from build123d import *

# Parameters (mm, degrees)
SKETCH_2_R          = 55
EXTRUDE_1_DEPTH     = 15
SKETCH_3_R          = 50
CUT_EXTRUDE_1_DEPTH = 10
EXTRUDE_3_DEPTH     = 15
CUT_EXTRUDE_4_DEPTH = 10
CUT_EXTRUDE_5_DEPTH = 10
FILLET_1_R          = 5
FILLET_2_R          = 5
FILLET_3_R          = 5


with BuildPart() as part:
    # 草圖2 → 填料-伸長1 (new body)
    with BuildSketch(Plane(origin=(0, 0, 0), x_dir=(1, 0, 0), z_dir=(0, 1, 0))):
        with Locations(Location((0, 0, 0), (0, 0, 270))):
            Circle(SKETCH_2_R)
    extrude(amount=EXTRUDE_1_DEPTH)

    # 草圖3 → 除料-伸長1 (cut)
    with BuildSketch(Plane(origin=(0, 15, 0), x_dir=(1, 0, 0), z_dir=(0, 1, 0))):
        with Locations(Location((0, 0, 0), (0, 0, 270))):
            Circle(SKETCH_3_R)
    extrude(amount=-CUT_EXTRUDE_1_DEPTH, mode=Mode.SUBTRACT)

    # 草圖8 → 填料-伸長3 (add)
    with BuildSketch(Plane.XZ):
        with BuildLine():
            ThreePointArc((55, 0), (23.675491822, -49.643439516), (-34.617130436, -42.739376228))
            ThreePointArc((-34.617130436, -42.739376228), (6.919661262, -68.581943503), (55, -77.605489076))
            Line((55, -77.605489076), (55, 0))
        make_face()
        with BuildLine():
            ThreePointArc((-55, 0), (-38.890872965, 38.890872965), (0, 55))
            Line((0, 55), (-55, 55))
            Line((-55, 55), (-55, 0))
        make_face()
    extrude(amount=-EXTRUDE_3_DEPTH)

    # 草圖9 → 除料-伸長4 (cut)
    with BuildSketch(Plane(origin=(0, 15, 0), x_dir=(1, 0, 0), z_dir=(0, 1, 0))):
        with BuildLine():
            ThreePointArc((-31.352560089, 38.948902113), (21.591340805, 45.097827023), (50, 0))
            Line((50, 0), (50, 72.507493279))
            ThreePointArc((50, 72.507493279), (6.339263066, 62.963102381), (-31.352560089, 38.948902113))
        make_face()
    extrude(amount=-CUT_EXTRUDE_4_DEPTH, mode=Mode.SUBTRACT)

    # 草圖10 → 除料-伸長5 (cut)
    with BuildSketch(Plane(origin=(0, 15, 0), x_dir=(1, 0, 0), z_dir=(0, 1, 0))):
        with BuildLine():
            Line((0, -50), (-50, -50))
            Line((-50, -50), (-50, 0))
            ThreePointArc((-50, 0), (-35.355339059, -35.355339059), (0, -50))
        make_face()
    extrude(amount=-CUT_EXTRUDE_5_DEPTH, mode=Mode.SUBTRACT)

    # 圓角1
    fillet_1_edges = [part.edges().sort_by_distance(p)[0] for p in [
        (-50, 10, 50),
    ]]
    fillet(fillet_1_edges, radius=FILLET_1_R)

    # 圓角2
    fillet_2_edges = [part.edges().sort_by_distance(p)[0] for p in [
        (50, 10, -72.507493279),
    ]]
    fillet(fillet_2_edges, radius=FILLET_2_R)

    # 圓角3
    fillet_3_edges = [part.edges().sort_by_distance(p)[0] for p in [
        (55, 7.5, -77.605489076),
        (-55, 7.5, 55),
    ]]
    fillet(fillet_3_edges, radius=FILLET_3_R)


solid = part.part
Input: part model. Units: mm. Frame: model coordinates. A direction names the side the tool comes from. Give positions to 0.01 mm unless a question says otherwise; leave off trailing zeros. Loops run counter-clockwise (first coordinate to the right, second up) from the corner with the lowest first, then second, coordinate; pieces in that order, holes last. Notation, with made-up numbers: M -39.5,27.25 L 2.5,27.25 A16 ccw 2.5,50.25 Z; hole C 51.25,-20 d9. An arc over 180 degrees is marked long. Use CSV: the item, a comma, the result in double quotes.
(1) Section C-C, the plane z = 19. Return loops of the section in (x, y), plus the area to 3 significant figures.
Outcome:
outline,"M -55,0 L 51.61,0 L 51.61,15 L 46.25,15 L 46.25,5 L -50,5 L -50,15 L -55,15 Z"
area,"637 mm²"
(2) Pull-direction query (Y, two-part tool) for faces 3 (the face through (-50, 10, 23)), 4 (the face through (-1, 0, -10)), 5 (the face through (-25, 15, -45)); classes: pulls with the +Y half, pulls with the -Y half, needs draft (parallel to the pull), parting line crosses it, or undercut.
Outcome:
face 3,"needs draft"
face 4,"pulls with the -Y half"
face 5,"pulls with the +Y half"
(3) Material intervals for L1, parallel to Y at x = -28.5, z = -37; L2, parallel to Z at x = -22.5, y = 7.25; L3, parallel to X at y = 9.75, z = -7, sorted ascending. Write a range as [from, to].
Outcome:
L1,"y = [0, 5]"
L2,"z = [-52.6, -46.38], [50, 55]"
L3,"x = [-54.55, -49.51], [50, 55]"
(4) Section A-A, the plane y = 8.25. Return loops of the section in (x, z), plus the area to 3 significant figures.
Outcome:
outline,"M -55,0 A55 ccw -34.62,-42.74 A132.61 ccw 49.8,-77.5 A5 ccw 55,-72.51 L 55,0 A55 ccw 0,55 L -50,55 A5 ccw -55,50 Z; hole M -50,0 A50 ccw -31.35,-38.95 A127.61 ccw 44.59,-72.18 A5 ccw 50,-67.2 L 50,0 A50 ccw 0,50 L -45,50 A5 ccw -50,45 Z"
area,"2,020 mm²"
(5) Set-up query: faces 1 (the face through (38.461, 7.395, 39.316)), 2 (the face through (-48, 10, 49)). Return all of +Z, -Z, +X, -X, +Y, -Y with unobstructed straight access to the full face (end or side cutting, diameter ignored); none if empty.
Outcome:
face 1,"+Z, +X, +Y, -Y"
face 2,"+Y"
(6) Pin query (flat end, axial travel): P1, Ø3, axis at x = -40, y = 4.5, coming from the -Z side; P2, Ø5, axis at x = -6.5, y = 3, coming from the -Z side; P3, Ø4, axis at x = 41.5, y = 7, coming from the +Z side. Return the tip coordinate at first contact, or that it passes through.
Outcome:
P1,"stops at z = -39.28"
P2,"stops at z = -63.76"
P3,"stops at z = 38.27"
(7) Section B-B, the plane x = -2. Return loops of the section in (y, z), plus the area to 3 significant figures.
Outcome:
outline,"M 0,-64.73 L 15,-64.73 L 15,-59.17 L 5,-59.17 L 5,50 L 15,50 L 15,55 L 0,55 Z"
area,"704 mm²"
